Could you check a few things on this model? Use its own coordinates, in mm. Give positions to 0.01 mm unless a question says otherwise; leave off trailing zeros. Order: outer loops, then holes, each group sorted by start corner. A loop starts at its lowest first (then second) coordinate and runs counter-clockwise, first axis right, second up.
from build123d import *

# Parameters (mm, degrees)
BOSS_EXTRUDE1_DEPTH = 10
SKETCH3_R           = 1.775
CUT_EXTRUDE2_DEPTH  = 163.750712068
SKETCH4_W           = 12
SKETCH4_H           = 10
BOSS_EXTRUDE2_DEPTH = 7
SKETCH5_R           = 2.479798403
CUT_EXTRUDE3_DEPTH  = 10
FILLET1_R           = 2
FILLET2_R           = 2


with BuildPart() as part:
    # Sketch1 → Boss-Extrude1 (new body)
    with BuildSketch(Plane.XY):
        Polygon((-79.341642805, -34.372803322), (-79.341642805, -44.372803322), (-121.341642805, -44.372803322), (-121.341642805, 73.627196678), (33.658357195, 73.627196678), (33.658357195, -44.372803322), (-8.341642805, -44.372803322), (-8.341642805, -34.372803322), (23.658357195, -34.372803322), (23.658357195, 63.627196678), (-111.341642805, 63.627196678), (-111.341642805, -34.372803322), align=None)
    extrude(amount=BOSS_EXTRUDE1_DEPTH)

    # Sketch3 → Cut-Extrude2 (cut, through all)
    with BuildSketch(Plane(origin=(0, -34.372803322, 0), x_dir=(1, 0, 0), z_dir=(0, 1, 0))):
        with Locations(Location((-84.841642805, -5, 0), (0, 0, 270))):
            Circle(SKETCH3_R)
        with Locations(Location((-2.841642805, -5, 0), (0, 0, 270))):
            Circle(SKETCH3_R)
    extrude(amount=-CUT_EXTRUDE2_DEPTH, mode=Mode.SUBTRACT)

    # Sketch4 → Boss-Extrude2 (add)
    with BuildSketch(Plane.XY.offset(10)):
        with Locations((-83.341642805, 68.627196678)):
            Rectangle(SKETCH4_W, SKETCH4_H)
        with Locations((-4.341642805, 68.627196678)):
            Rectangle(SKETCH4_W, SKETCH4_H)
    extrude(amount=BOSS_EXTRUDE2_DEPTH)

    # Sketch5 → Cut-Extrude3 (cut)
    with BuildSketch(Plane(origin=(0, 73.627196678, 0), x_dir=(1, 0, 0), z_dir=(0, 1, 0))):
        with Locations(Location((-83.341642805, -11.5, 0), (0, 0, 270))):
            Circle(SKETCH5_R)
        with Locations(Location((-4.341642805, -11.5, 0), (0, 0, 270))):
            Circle(SKETCH5_R)
    extrude(amount=-CUT_EXTRUDE3_DEPTH, mode=Mode.SUBTRACT)

    # Fillet1
    fillet1_edges = [part.edges().sort_by_distance(p)[0] for p in [
        (-77.341642805, 68.627196678, 17),
        (-89.341642805, 68.627196678, 17),
    ]]
    fillet(fillet1_edges, radius=FILLET1_R)

    # Fillet2
    fillet2_edges = [part.edges().sort_by_distance(p)[0] for p in [
        (-10.341642805, 68.627196678, 17),
        (1.658357195, 68.627196678, 17),
    ]]
    fillet(fillet2_edges, radius=FILLET2_R)


solid = part.part
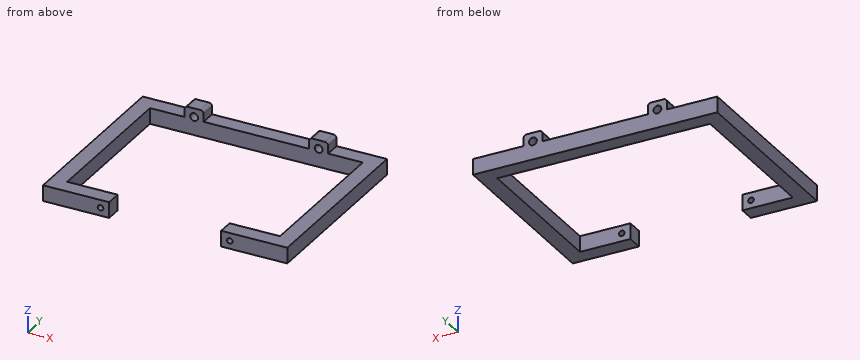
Item 1: Please list where these lines run through material, in increasing order: line 1 along X through (y, z) = (-40.25, 5); line 2 along X through (y, z) = (-16, 6.25); line 3 along Y through (x, z) = (-105.5, 1.75).
Findings:
line 1: x = -121.34 to -86.62, -83.07 to -79.34, -8.34 to -4.62, -1.07 to 33.66
line 2: x = -121.34 to -111.34, 23.66 to 33.66
line 3: y = -44.37 to -34.37, 63.63 to 73.63
Item 2: Imagine slicing it at C-C on z = 5. List the corners of the cut face in (x, y) for me.
Findings:
outline: (-121.34, -44.37) - (-86.62, -44.37) - (-86.62, -34.37) - (-111.34, -34.37) - (-111.34, 63.63) - (23.66, 63.63) - (23.66, -34.37) - (-1.07, -34.37) - (-1.07, -44.37) - (33.66, -44.37) - (33.66, 73.63) - (-121.34, 73.63) - close; (-83.07, -44.37) - (-79.34, -44.37) - (-79.34, -34.37) - (-83.07, -34.37) - close; (-8.34, -44.37) - (-4.62, -44.37) - (-4.62, -34.37) - (-8.34, -34.37) - close
Item 3: Imagine slicing it at D-D on x = -30.5. List the corners of the cut face in (y, z) for me, then the cut area to 3 significant figures.
Findings:
outline: (63.63, 0) - (73.63, 0) - (73.63, 10) - (63.63, 10) - close
area: 100 mm2
Item 4: Imagine slicing it at A-A on x = 11. List the corners of the cut face in (y, z) for me, then the cut area to 3 significant figures.
Findings:
outline: (-44.37, 0) - (-34.37, 0) - (-34.37, 10) - (-44.37, 10) - close; (63.63, 0) - (73.63, 0) - (73.63, 10) - (63.63, 10) - close
area: 200 mm2
Item 5: Imagine slicing it at B-B on y = 9. List the corners of the cut face in (x, z) for me.
Findings:
outline: (-121.34, 0) - (-111.34, 0) - (-111.34, 10) - (-121.34, 10) - close; (23.66, 0) - (33.66, 0) - (33.66, 10) - (23.66, 10) - close
Item 6: For pin 1 (3 mm diameter, centred on x = -1, z = 12.5, fed in from -Y); pin 2 (2.5 mm diameter, centred on y = 70, z = 12.5, fed in from +X), each with a flat end and sliding along its axis, tell me the tip position at first contact or that it passes through.
Findings:
pin 1: stops at y = 63.63
pin 2: stops at x = 1.66
